```python
from build123d import *

# Parameters (mm, degrees)
BOSS_EXTRUDE1_DEPTH      = 7.25
BOSS_EXTRUDE1_DEPTH_BACK = 7.25
SKETCH2_W                = 0.675
SKETCH2_H                = 6
SKETCH2_W_2              = 2.5
SKETCH2_H_2              = 7.8
CUT_EXTRUDE1_DEPTH       = 24.646617094
SKETCH3_W                = 5
SKETCH3_H                = 6
CUT_EXTRUDE2_DEPTH       = 8.2
SKETCH4_R                = 1.75
CUT_EXTRUDE3_DEPTH       = 24.646617094


with BuildPart() as part:
    # Sketch1 → Boss-Extrude1 (new, two sides: drawn at the far end of the back side and taken through both)
    with BuildSketch(Plane(origin=(0, 0, 0), x_dir=(0, 0, -1), z_dir=(1, 0, 0)).offset(-BOSS_EXTRUDE1_DEPTH_BACK)):
        Polygon((-15.5, 0), (15.5, 0), (15.5, 5.65), (20.8, 5.65), (20.8, 6.3), (13, 6.3), (13, 3), (-9.5, 3), (-9.5, 11.6), (-15.5, 11.6), align=None)
    extrude(amount=BOSS_EXTRUDE1_DEPTH + BOSS_EXTRUDE1_DEPTH_BACK)

    # Sketch2 → Cut-Extrude1 (cut, through all)
    with BuildSketch(Plane(origin=(0, 3, 0), x_dir=(1, 0, 0), z_dir=(0, 1, 0))):
        with Locations((-6.9125, -12.5)):
            Rectangle(SKETCH2_W, SKETCH2_H)
        with Locations((6.9125, -12.5)):
            Rectangle(SKETCH2_W, SKETCH2_H)
        with Locations((6, 16.9)):
            Rectangle(SKETCH2_W_2, SKETCH2_H_2)
        with Locations((-6, 16.9)):
            Rectangle(SKETCH2_W_2, SKETCH2_H_2)
    extrude(amount=CUT_EXTRUDE1_DEPTH, mode=Mode.SUBTRACT)

    # Sketch3 → Cut-Extrude2 (cut)
    with BuildSketch(Plane(origin=(0, 11.6, 0), x_dir=(1, 0, 0), z_dir=(0, 1, 0))):
        with Locations((0, -12.5)):
            Rectangle(SKETCH3_W, SKETCH3_H)
    extrude(amount=-CUT_EXTRUDE2_DEPTH, mode=Mode.SUBTRACT)

    # Sketch4 → Cut-Extrude3 (cut, through all)
    with BuildSketch(Plane(origin=(0, 3, 0), x_dir=(1, 0, 0), z_dir=(0, 1, 0))):
        with Locations(Location((0, 7.95, 0), (0, 0, 270))):
            Circle(SKETCH4_R)
    extrude(amount=-CUT_EXTRUDE3_DEPTH, mode=Mode.SUBTRACT)


solid = part.part
```
Part model, mm, in its own coordinate system. A direction names the side the tool comes from. Give positions to 0.01 mm unless a question says otherwise; leave off trailing zeros. Write each loop counter-clockwise with the first axis right and the second up, starting at its lowest first coordinate (ties: lowest second). Pieces come first, ordered by that corner, then holes. Notation, with made-up numbers: (2, 55) -> (12, 55) arc R21 ccw to (12, 89) -> close; hole circle Ø6 at (69.25, 88). An arc over 180 degrees is marked (long way). Put each result on its own line as item: value. Start each with the question number.
Item 1: Cut at B-B (y = 4). List the corners of the cut face in (x, z) (3 decimals), then the cut area to 4 significant figures.
Item 2: Pull direction X, two halves, no side cores. Call faces 4 (the face through (-6.575, 7, 13)), 5 (the face through (6.575, 7, 13)), 6 (the face through (-0.67, 1.521, -6.333)): pulls with the +X half, pulls with the -X half, needs draft (parallel to the pull), parting line crosses it, or undercut.
Item 3: Pin check, flat tips, straight feed: pin 1 Ø5 at (y, z) = (7, 11) entering from -X (3 decimals); pin 2 Ø4.5 at (x, y) = (1.5, 2.5) entering from -Z; pin 3 Ø2.5 at (x, z) = (1.5, -17.5) entering from +Y. Stop position of each tip, or through.
Item 4: Cut at D-D (y = 6.75). List the corners of the cut face in (x, z) (3 decimals), then the cut area to 3 significant figures.
Item 5: Cut at A-A (x = 0). List the corners of the cut face in (y, z).
Item 6: Wall check: L1, parallel to X at y = 8, z = 11.5 (3 decimals); L2, parallel to X at y = 2.1, z = -7.95; L3, parallel to Z at x = 4.5, y = 1.5. Give the ranges that are in metal, low to high. Write a range as [from, to].
Item 7: Which spindle directions (+Z, -Z, +X, -X, +Y, -Y) get a long thin tool onto all of the face, cutting with end or side? Do faces 1 (the face through (2.5, 8, 13)), 2 (the face through (0, 6.3, -17)), 3 (the face through (-3, 7, 9.5)). Say none if no direction does.
Item 8: Cut at C-C (z = -7.95). List the corners of the cut face in (x, y).
Answer list:
1. outline: (-6.575, 9.5) -> (-2.5, 9.5) -> (-2.5, 15.5) -> (-6.575, 15.5) -> close; (-4.75, -15.5) -> (4.75, -15.5) -> (4.75, -13) -> (-4.75, -13) -> close; (2.5, 9.5) -> (6.575, 9.5) -> (6.575, 15.5) -> (2.5, 15.5) -> close
1. area: 72.65 mm2
2. face 4: pulls with the -X half
2. face 5: pulls with the +X half
2. face 6: undercut
3. pin 1: stops at x = -6.575
3. pin 2: stops at z = -15.5
3. pin 3: stops at y = 6.3
4. outline: (-6.575, 9.5) -> (-2.5, 9.5) -> (-2.5, 15.5) -> (-6.575, 15.5) -> close; (2.5, 9.5) -> (6.575, 9.5) -> (6.575, 15.5) -> (2.5, 15.5) -> close
4. area: 48.9 mm2
5. outline: (0, -15.5) -> (5.65, -15.5) -> (5.65, -20.8) -> (6.3, -20.8) -> (6.3, -13) -> (3, -13) -> (3, -9.7) -> (0, -9.7) -> close; (0, -6.2) -> (3, -6.2) -> (3, 9.5) -> (3.4, 9.5) -> (3.4, 15.5) -> (0, 15.5) -> close
6. L1: x = [-6.575, -2.5], [2.5, 6.575]
6. L2: x = [-7.25, -1.75], [1.75, 7.25]
6. L3: z = [-15.5, 15.5]
7. face 1: +Z, +Y
7. face 2: -Z, +X, -X, +Y
7. face 3: +X, -X, +Y
8. outline: (-7.25, 0) -> (-1.75, 0) -> (-1.75, 3) -> (-7.25, 3) -> close; (1.75, 0) -> (7.25, 0) -> (7.25, 3) -> (1.75, 3) -> close
